Autodesk Inventor part; units mm, degrees
ref_plane "YZ Plane" through (0, 0, 0) normal (1, 0, 0) x (0, 1, 0)
ref_plane "XZ Plane" through (0, 0, 0) normal (0, 1, 0) x (-1, 0, 0)
ref_plane "XY Plane" through (0, 0, 0) normal (0, 0, 1) x (1, 0, 0)
ref_plane "作業平面1" through (0, 0, 0) normal (0, 0, 1) x (1, 0, 0)
sketch "スケッチ2" plane through (0, 0, 0) normal (0, 0, 1) x (1, 0, 0)
  line L0 (110, -57) -> (-40, -57)
  line L1 (-40, -57) -> (-40, -93)
  line L2 (-40, -93) -> (110, -93)
  line L3 (110, -93) -> (110, -57)
  circle A0 centre (0, -75) radius 6 construction
  circle A1 centre (0, -75) radius 75 construction
  point P0 (0, 0)
  dimension "d1" = 150
  dimension "d2" = 18
  dimension "d3" = 18
  dimension "d4" = 40
  dimension "d29" = 110
extrude "押し出し1" add sketch "スケッチ2" along normal blind 3
sketch "スケッチ3" plane through (0, 0, 3) normal (0, 0, 1) x (1, 0, 0)
  circle A0 centre (0, -75) radius 6 construction
  circle A1 centre (0, -75) radius 7
  line L0 (0, -68) -> (-38.1, -68) construction
  line L1 (-38.1, -68) -> (-38.1, -82) construction
  line L2 (-38.1, -82) -> (0, -82) construction
  line L3 (0, -82) -> (0, -68) construction
  line L4 (0, -68) -> (-40, -68)
  line L5 (-40, -68) -> (-40, -82)
  line L6 (-40, -82) -> (0, -82)
  line L7 (0, -82) -> (0, -68)
  line L8 (-40, -57) -> (-40, -93)
  point P0 (0, 0)
  point P1 (0, -82)
  dimension "d8" = 14
extrude "押し出し2" cut sketch "スケッチ3" against normal blind 14
fillet "フィレット1" radius 10 2 edges at (-40, -68, 1.5) (-40, -82, 1.5)
ref_plane "作業平面2" through (-40, -75, 0) normal (0, -1, 0) x (1, 0, 0)
sketch "スケッチ4" plane through (0, 0, 3) normal (0, 0, 1) x (1, 0, 0)
  line L0 (-40, -93) -> (110, -93)
  line L1 (110, -57) -> (-40, -57)
  line L2 (110, -93) -> (110, -57)
  point P0 (0, 0)
  point P1 (95, -75)
  dimension "d25" = 15
  dimension "d26" = 36
  dimension "d27" = 18
hole "穴1" at (95, -75, 3) direction (0, 0, -1) diameter 6.6 end through all
fillet "フィレット2" radius 5 2 edges at (110, -57, 1.5) (110, -93, 1.5)
fillet "フィレット2" radius 2 2 edges at (-40, -57, 1.5) (-40, -93, 1.5)
equation "\"d3\" = d2"
equation "\"d9\" = d8"
properties part number "wheel_mount" material "アルミニウム 6061"
Model file for the job. Use its own axes, mm. A direction names the side the tool comes from. Give positions to 0.01 mm unless a question says otherwise; leave off trailing zeros. Order: outer loops, then holes, each group sorted by start corner. A loop starts at its lowest first (then second) coordinate and runs counter-clockwise, first axis right, second up.
1) Mould opens along Y. For faces 3 (the flat face through (-15, -82, 2)), 4 (the flat face through (33, -93, 1)), 5 (the cylindrical face through (92.77, -72.57, 1.48)), 6 (the cylindrical face through (109, -59, 2)) say: +Y half, -Y half, draft (parallel to the pull), parting line (faces both ways), or undercut.
2) Saw through at A-A, the plane y = -75. Write the cut outline in (x, z), then the cut area to 3 significant figures.
3) 3-axis set-ups, long thin cutter, end or side, ignore diameter. For faces 1 (the cylindrical face through (-36.5, -65.6, 1.5)), 2 (the flat face through (34, -75, 3)): which of +Z, -Z, +X, -X, +Y, -Y reach the whole face in a straight line?
4) Saw through at C-C, the plane y = -83.5. Write the cut outline in (x, z), then the cut area to 3 significant figures.
5) Pin check, flat tip, straight feed: pin 1 (1.5 mm diameter, centred on y = -70.5, z = 1.5, fed in from -X). Stop position of the tip, or through.
6) Saw through at D-D, the plane y = -69.5. Write the cut outline in (x, z).
7) Saw through at B-B, the plane x = 95. Write the cut outline in (y, z).
8) Wall check: probe 1 along X at (y, z) = (-75, 1.5); probe 2 along Y at (x, z) = (-11.5, 2.95); probe 3 along Y at (x, z) = (95, 1.8). Give the ranges that are in metal, low to high.
Computed:
1. face 3: undercut
1. face 4: -Y half
1. face 5: undercut
1. face 6: +Y half
2. outline: (7, 0) - (91.7, 0) - (91.7, 3) - (7, 3) - close; (98.3, 0) - (110, 0) - (110, 3) - (98.3, 3) - close
2. area: 289 mm2
3. face 1: +Z, -Z, -X
3. face 2: +Z, +X, -X, +Y, -Y
4. outline: (-35.27, 0) - (110, 0) - (110, 3) - (-35.27, 3) - close
4. area: 436 mm2
5. pin 1: stops at x = 4.63
6. outline: (4.33, 0) - (110, 0) - (110, 3) - (4.33, 3) - close
7. outline: (-93, 0) - (-78.3, 0) - (-78.3, 3) - (-93, 3) - close; (-71.7, 0) - (-57, 0) - (-57, 3) - (-71.7, 3) - close
8. probe 1: x = 7 to 91.7, 98.3 to 110
8. probe 2: y = -93 to -82, -68 to -57
8. probe 3: y = -93 to -78.3, -71.7 to -57
